from build123d import *

# Parameters (mm, degrees)
ESQUISSE1_W        = 46
ESQUISSE1_H        = 46
BOSS_EXTRU_1_DEPTH = 38
ESQUISSE2_R        = 7.25
BOSS_EXTRU_2_DEPTH = 17


with BuildPart() as part:
    # Esquisse1 → Boss.-Extru.1 (new body)
    with BuildSketch(Plane(origin=(0, 0, 0), x_dir=(1, 0, 0), z_dir=(0, 1, 0))):
        with Locations((-54.433333333, 4.063333333)):
            Rectangle(ESQUISSE1_W, ESQUISSE1_H)
    extrude(amount=BOSS_EXTRU_1_DEPTH)

    # Esquisse2 → Boss.-Extru.2 (add)
    with BuildSketch(Plane(origin=(0, 38, 0), x_dir=(1, 0, 0), z_dir=(0, 1, 0))):
        with Locations(Location((-55.433333333, 4.563333333, 0), (0, 0, 270))):
            Circle(ESQUISSE2_R)
    extrude(amount=BOSS_EXTRU_2_DEPTH)


solid = part.part
The listing builds one solid part. Answer for the finished solid, in the listing's coordinates (mm). A direction names the side the tool comes from. Coordinates: 2 decimals unless noted, no trailing zeros. Loops run counter-clockwise (first coordinate to the right, second up) from the corner with the lowest first, then second, coordinate; pieces in that order, holes last. Notation, with made-up numbers: (57.25, -26) -> (98.25, -26) arc R34 cw to (98.25, 13) -> close; hole circle Ø10 at (-37, -31). An arc over 180 degrees is marked (long way). Answer in a Markdown table with one row per item. Add a question column.
1. Consider line 1 (Y direction, x = -34.5, z = 5); line 2 (X direction, y = 46.5, z = -9); line 3 (X direction, y = 39, z = -2.5). Determine where each line is inside the solid, lowest interval first. Write a range as [from, to].
2. Flat-ended cylindrical pins translate along their axes: P1, Ø6, axis at x = -54.5, z = 6, coming from the +Y side; P2, Ø6, axis at x = -42, z = -10, coming from the -Y side. Find the tip coordinate at first contact, or state that the pin passes through.
3. The part is cut by section D-D, the plane z = -3. Write down the section's boundary in (x, y).
4. For faces 1 (the flat face through (-49.6, 38, -9.5)), 2 (the flat face through (-55, 19, 18.937)), determine the directions among +Z, -Z, +X, -X, +Y, -Y from which every point of the face is accessible in a straight line to the end or side of a thin tool.
5. The part is cut by section A-A, the plane z = -8. Write down the section's boundary in (x, y).
6. The part is cut by section B-B, the plane x = -64.5. Write down the section's boundary in (y, z).
7. The part is cut by section C-C, the plane y = 50. Write down the section's boundary in (x, z).
Answer below:
| question | item | result |
|---|---|---|
| 1 | line 1 | [0, 38] |
| 1 | line 2 | [-61.17, -49.7] |
| 1 | line 3 | [-62.38, -48.48] |
| 2 | P1 | y = 38 |
| 2 | P2 | y = 0 |
| 3 | outline | (-77.43, 0) -> (-31.43, 0) -> (-31.43, 38) -> (-48.35, 38) -> (-48.35, 55) -> (-62.51, 55) -> (-62.51, 38) -> (-77.43, 38) -> close |
| 4 | face 1 | +Y |
| 4 | face 2 | +Z, +X, -X, +Y, -Y |
| 5 | outline | (-77.43, 0) -> (-31.43, 0) -> (-31.43, 38) -> (-49.05, 38) -> (-49.05, 55) -> (-61.82, 55) -> (-61.82, 38) -> (-77.43, 38) -> close |
| 6 | outline | (0, -27.06) -> (38, -27.06) -> (38, 18.94) -> (0, 18.94) -> close |
| 7 | outline | circle Ø14.5 at (-55.43, -4.56) |
